from build123d import *

# Parameters (mm, degrees)
F1_DEPTH = 4
F2_SIZE  = 2
F4_DEPTH = 15
F4_TAPER = -4


with BuildPart() as f1:
    # F0 (on Top) → F1 (new body)
    with BuildSketch(Plane.XY):
        Polygon((5, -30), (5, -5), (30, -5), (30, 5), (5, 5), (5, 30), (-5, 30), (-5, 5), (-30, 5), (-30, -5), (-5, -5), (-5, -30), align=None)
    extrude(amount=F1_DEPTH)

    # F2
    f2_edges = [f1.edges().sort_by_distance(p)[0] for p in [
        (-5, 17.5, 4),
        (0, 30, 4),
        (5, 17.5, 4),
        (-17.5, 5, 4),
        (-17.5, -5, 4),
        (-30, 0, 4),
        (-5, -17.5, 4),
        (0, -30, 4),
        (5, -17.5, 4),
        (17.5, -5, 4),
        (17.5, 5, 4),
        (30, 0, 4),
    ]]
    chamfer(f2_edges, length=F2_SIZE)

    # F3 (on face) → F4 (join)
    with BuildSketch(Plane.XY.offset(4)):
        with BuildLine():
            ThreePointArc((3, -3), (3.9196888946, -1.6235883004), (4.2426406871, 0))
            ThreePointArc((4.2426406871, 0), (3.9196888946, 1.6235883004), (3, 3))
            ThreePointArc((3, 3), (0, 4.2426406871), (-3, 3))
            ThreePointArc((-3, 3), (-4.2426406871, 0), (-3, -3))
            ThreePointArc((-3, -3), (0, -4.2426406871), (3, -3))
        make_face()
    extrude(amount=F4_DEPTH, taper=F4_TAPER)


solid = f1.part
The model under review builds one solid part; all positions refer to its coordinate system, in mm. A direction names the side the tool comes from. Give positions to 0.01 mm unless a question says otherwise; leave off trailing zeros. Loops run counter-clockwise (first coordinate to the right, second up) from the corner with the lowest first, then second, coordinate; pieces in that order, holes last. Notation, with made-up numbers: (20, 60) -> (67, 60) arc R16 ccw to (67, 81) -> close; hole circle Ø5 at (32.25, 78). An arc over 180 degrees is marked (long way). Put each result on its own line as item: value. Start each with the question number.
1. For faces 1 (the face through (-5, -17, 1)), 2 (the face through (0, -29, 3)), list the 3-axis set-ups (+Z, -Z, +X, -X, +Y, -Y) from which the entire face can be reached by the end or side of a thin tool; tool diameter is ignored.
2. Wall thickness on probe 1 along Z at (x, y) = (1, -18); probe 2 along X at (y, z) = (-7, 3.25); probe 3 along Y at (x, z) = (11, 1.5): over which ranges is each line inside the solid? List them lowest first.
3. We need section A-A on x = 26.5. State the section outline as (y, z) points, then the cut area to 3 significant figures.
4. Clearance check with flat-ended pins moving along their axes: P1, Ø2, axis at x = -12.5, z = 1, coming from the +Y side; P2, Ø0.6, axis at x = -22.5, z = 1, coming from the -Y side; P3, Ø2, axis at x = -4, z = 5, coming from the +Y side; P4, Ø6, axis at x = 19.5, y = 9, coming from the +Z side. State where each tip first meets the part, or that it passes through.
Determined:
1. face 1: +Z, -Z, -X, -Y
1. face 2: +Z, +X, -X, -Y
2. probe 1: 0 to 4
2. probe 2: -3.75 to 3.75
2. probe 3: -5 to 5
3. outline: (-5, 0) -> (5, 0) -> (5, 2) -> (3, 4) -> (-3, 4) -> (-5, 2) -> close
3. area: 36.0 mm^2
4. P1: y = 5
4. P2: y = -5
4. P3: y = 3.1
4. P4: through
